```python
from build123d import *

# Parameters (mm, degrees)
SKETCH1_W                   = 173.0375
SKETCH1_H                   = 114.3
BOSS_EXTRUDE1_DEPTH         = 3.175
SKETCH3_R                   = 3.175
SKETCH3_R_2                 = 3.7703125
CUT_EXTRUDE1_DEPTH          = 4.175
F_6_CLEARANCE_HOLE1_D       = 4.3053
F_2_CLEARANCE_HOLE1_D       = 2.7051
SKETCH8_W                   = 58.74
SKETCH8_H                   = 26.99
CUT_EXTRUDE2_DEPTH          = 4.175
F_3_0_213_DIAMETER_HOLE1_D  = 5.4102
F_3_0_3_DIAMETER_HOLE1_D    = 3
FILLET1_R                   = 1.27
FILLET2_R                   = 2.54
F_1_4_CLEARANCE_HOLE1_D     = 7.14248
F_1_4_CLEARANCE_HOLE1_DEPTH = 3.175
CUT_EXTRUDE3_REACH          = 5.175
SKETCH14_W                  = 3.175
SKETCH14_H                  = 15.875
FILLET3_R                   = 1.5875
FILLET4_R                   = 2.54
CUT_EXTRUDE4_START          = -3.175
SKETCH15_W                  = 65.7
SKETCH15_H                  = 26.99
CUT_EXTRUDE4_DEPTH          = 3.175
CUT_EXTRUDE5_REACH          = 5.175
SKETCH16_R                  = 1.190625


with BuildPart() as part:
    # Sketch1 → Boss-Extrude1 (new body)
    with BuildSketch(Plane.XY):
        with Locations((25.118, -40.513)):
            Rectangle(SKETCH1_W, SKETCH1_H)
    extrude(amount=BOSS_EXTRUDE1_DEPTH)

    # Sketch3 → Cut-Extrude1 (cut, through all)
    with BuildSketch(Plane.XY.offset(3.175)):
        with Locations((100.302, -26.543)):
            Circle(SKETCH3_R)
        with Locations((99.413, -51.6255)):
            Circle(SKETCH3_R_2)
        with Locations((-47.907, -51.6255)):
            Circle(SKETCH3_R_2)
        with Locations((-47.907, -6.5405)):
            Circle(SKETCH3_R_2)
    extrude(amount=-CUT_EXTRUDE1_DEPTH, mode=Mode.SUBTRACT)

    # #6 Clearance Hole1 (through all)
    with Locations(Plane.XY.offset(3.175)):
        with Locations((18.387, 10.287), (-56.162, -40.894), (106.398, -40.894), (18.387, -91.313)):
            Hole(F_6_CLEARANCE_HOLE1_D / 2)

    # #2 Clearance Hole1 (through all)
    with Locations(Plane.XY.offset(3.175)):
        with Locations((26.788, 12.7), (89.488, 12.7), (89.488, -18.6), (26.788, -18.6)):
            Hole(F_2_CLEARANCE_HOLE1_D / 2)

    # Sketch8 → Cut-Extrude2 (cut, through all)
    with BuildSketch(Plane.XY.offset(3.175)):
        with Locations((58.138, -3.125)):
            Rectangle(SKETCH8_W, SKETCH8_H)
        Polygon((14.64685, 6.54685), (14.64685, 10.287), (-41.367, 10.287), (-41.367, -13.0805), (-55.05075, -13.0805), (-55.05075, -35.56635), (-50.83435, -35.56635), (-50.83435, -45.0855), (-41.367, -45.0855), (-41.367, -58.1655), (-55.05075, -58.1655), (-55.05075, -91.313), (13.05935, -91.313), (13.05935, -88.138), (105.28675, -88.138), (105.28675, -58.1655), (92.658, -58.1655), (92.658, -45.0855), (101.07035, -45.0855), (101.07035, -32.150898303), (92.658, -32.150898303), (92.658, -23.12755), (22.26045, -23.12755), (22.26045, 6.54685), align=None)
    extrude(amount=-CUT_EXTRUDE2_DEPTH, mode=Mode.SUBTRACT)

    # #3 (0.213) Diameter Hole1 (through all)
    with Locations(Plane(origin=(18.387, 10.287, 3.175), x_dir=(1, 0, 0), z_dir=(0, 0, 1))):
        with Locations((0, 0), (-74.549, -51.181), (0, -101.6), (88.011, -51.181)):
            Hole(F_3_0_213_DIAMETER_HOLE1_D / 2)

    # Ø3.0 (3) Diameter Hole1 (through all)
    with Locations(Plane.XY.offset(3.175)):
        with Locations((26.788, 12.7), (89.488, 12.7), (89.488, -18.6), (26.788, -18.6)):
            Hole(F_3_0_3_DIAMETER_HOLE1_D / 2)

    # Fillet1
    fillet1_edges = [part.edges().sort_by_distance(p)[0] for p in [
        (14.64685, 10.287, 1.5875),
        (14.64685, 6.54685, 1.5875),
        (22.26045, 6.54685, 1.5875),
        (22.26045, -23.12755, 1.5875),
        (92.658, -23.12755, 1.5875),
        (92.658, -32.150898303, 1.5875),
        (101.07035, -32.150898303, 1.5875),
        (101.07035, -45.0855, 1.5875),
        (92.658, -45.0855, 1.5875),
        (92.658, -58.1655, 1.5875),
        (105.28675, -58.1655, 1.5875),
        (13.05935, -91.313, 1.5875),
        (-55.05075, -91.313, 1.5875),
        (-55.05075, -58.1655, 1.5875),
        (-41.367, -58.1655, 1.5875),
        (-41.367, -45.0855, 1.5875),
        (-50.83435, -45.0855, 1.5875),
        (-55.05075, -35.56635, 1.5875),
        (-55.05075, -13.0805, 1.5875),
        (-41.367, -13.0805, 1.5875),
        (-41.367, 10.287, 1.5875),
    ]]
    fillet(fillet1_edges, radius=FILLET1_R)

    # Fillet2
    fillet2_edges = [part.edges().sort_by_distance(p)[0] for p in [
        (13.05935, -88.138, 1.5875),
        (-50.83435, -35.56635, 1.5875),
        (111.63675, 16.637, 1.5875),
        (111.63675, -97.663, 1.5875),
        (-61.40075, -97.663, 1.5875),
        (-61.40075, 16.637, 1.5875),
    ]]
    fillet(fillet2_edges, radius=FILLET2_R)

    # 1/4 Clearance Hole1
    with Locations(Plane(origin=(0, 0, 0), x_dir=(-1, 0, 0), z_dir=(0, 0, -1))):
        with Locations((-102.7785, 10.287), (52.5425, 10.287)):
            Hole(F_1_4_CLEARANCE_HOLE1_D / 2, depth=F_1_4_CLEARANCE_HOLE1_DEPTH)

    # Sketch14 → Cut-Extrude3 (cut, up to next)
    with BuildSketch(Plane(origin=(0, 0, 0), x_dir=(-1, 0, 0), z_dir=(0, 0, -1)), mode=Mode.PRIVATE) as cut_extrude3_sk1:
        with Locations((-110.04925, 8.6995)):
            Rectangle(SKETCH14_W, SKETCH14_H)
    cut_extrude3_tool1 = extrude(cut_extrude3_sk1.sketch, amount=-CUT_EXTRUDE3_REACH, mode=Mode.PRIVATE) & part.part
    add(cut_extrude3_tool1.solids().sort_by_distance((110.04925, 8.6995, 0))[0], mode=Mode.SUBTRACT)
    # Sketch14 → Cut-Extrude3 (cut, up to next)
    with BuildSketch(Plane(origin=(0, 0, 0), x_dir=(-1, 0, 0), z_dir=(0, 0, -1)), mode=Mode.PRIVATE) as cut_extrude3_sk2:
        with Locations((59.81325, 8.6995)):
            Rectangle(SKETCH14_W, SKETCH14_H)
    cut_extrude3_tool2 = extrude(cut_extrude3_sk2.sketch, amount=-CUT_EXTRUDE3_REACH, mode=Mode.PRIVATE) & part.part
    add(cut_extrude3_tool2.solids().sort_by_distance((-59.81325, 8.6995, 0))[0], mode=Mode.SUBTRACT)

    # Fillet3
    fillet3_edges = [part.edges().sort_by_distance(p)[0] for p in [
        (108.46175, 0.762, 1.5875),
        (-58.22575, 0.762, 1.5875),
    ]]
    fillet(fillet3_edges, radius=FILLET3_R)

    # Fillet4
    fillet4_edges = [part.edges().sort_by_distance(p)[0] for p in [
        (111.63675, 0.762, 1.5875),
        (108.46175, 16.637, 1.5875),
        (-58.22575, 16.637, 1.5875),
        (-61.40075, 0.762, 1.5875),
    ]]
    fillet(fillet4_edges, radius=FILLET4_R)

    # Sketch15 → Cut-Extrude4 (cut)
    with BuildSketch(Plane(origin=(0, 0, 0), x_dir=(-1, 0, 0), z_dir=(0, 0, -1)).offset(CUT_EXTRUDE4_START)):
        with Locations((-58.138, -3.125)):
            Rectangle(SKETCH15_W, SKETCH15_H)
    extrude(amount=CUT_EXTRUDE4_DEPTH, mode=Mode.SUBTRACT)

    # Sketch16 → Cut-Extrude5 (cut, up to next)
    with BuildSketch(Plane(origin=(0, 0, 0), x_dir=(-1, 0, 0), z_dir=(0, 0, -1)), mode=Mode.PRIVATE) as cut_extrude5_sk1:
        with Locations((-98.142490655, -57.489441166)):
            Circle(SKETCH16_R)
    cut_extrude5_tool1 = extrude(cut_extrude5_sk1.sketch, amount=-CUT_EXTRUDE5_REACH, mode=Mode.PRIVATE) & part.part
    add(cut_extrude5_tool1.solids().sort_by_distance((98.142491, -57.489441, 0))[0], mode=Mode.SUBTRACT)
    # Sketch16 → Cut-Extrude5 (cut, up to next)
    with BuildSketch(Plane(origin=(0, 0, 0), x_dir=(-1, 0, 0), z_dir=(0, 0, -1)), mode=Mode.PRIVATE) as cut_extrude5_sk2:
        with Locations((49.177509345, -57.489441166)):
            Circle(SKETCH16_R)
    cut_extrude5_tool2 = extrude(cut_extrude5_sk2.sketch, amount=-CUT_EXTRUDE5_REACH, mode=Mode.PRIVATE) & part.part
    add(cut_extrude5_tool2.solids().sort_by_distance((-49.177509, -57.489441, 0))[0], mode=Mode.SUBTRACT)
    # Sketch16 → Cut-Extrude5 (cut, up to next)
    with BuildSketch(Plane(origin=(0, 0, 0), x_dir=(-1, 0, 0), z_dir=(0, 0, -1)), mode=Mode.PRIVATE) as cut_extrude5_sk3:
        with Locations((49.177509345, -12.404441166)):
            Circle(SKETCH16_R)
    cut_extrude5_tool3 = extrude(cut_extrude5_sk3.sketch, amount=-CUT_EXTRUDE5_REACH, mode=Mode.PRIVATE) & part.part
    add(cut_extrude5_tool3.solids().sort_by_distance((-49.177509, -12.404441, 0))[0], mode=Mode.SUBTRACT)


solid = part.part
```
For this review, take the finished solid that the model builds, in its own axes (mm). A direction names the side the tool comes from. Round coordinates to 2 decimals unless told otherwise and drop trailing zeros. Loops run counter-clockwise (first coordinate to the right, second up) from the corner with the lowest first, then second, coordinate; pieces in that order, holes last.
Q1. Mouldability with a two-part tool opening along X and no side actions: class faces 1 (the face through (58, -16.62, 2)), 2 (the face through (111.637, -49, 2)), 3 (the face through (24, 16.637, 2)) as +X half, -X half, draft (parallel to the pull), parting line (faces both ways), or undercut.
Result sheet:
face 1: undercut
face 2: +X half
face 3: draft
Q2. To check wall thickness, follow line 1 along Y through (x, z) = (81.5, 1.75); line 2 along X through (y, z) = (-1.5, 0.3); line 3 along X through (y, z) = (-40.5, 0.6). State the ranges of each line that lie inside material, in increasing order.
Result sheet:
line 1: y = -97.66 to -88.14, -23.13 to -16.62, 10.37 to 16.64
line 2: x = -61.4 to -41.37, 22.26 to 25.29, 90.99 to 111.63
line 3: x = -61.4 to -58.84, -53.49 to -50.83, 101.07 to 103.72, 109.07 to 111.64
Q3. Insertion check: pin 1 Ø1.4 at (x, y) = (-49.18, -57.49) entering from +Z (1 decimal). The pin has a flat end and moves straight along its axis. Give the tip position at first contact, or say it passes through.
Result sheet:
pin 1: passes through
Q4. Add section C-C on z = 0.7. Give the number of separate pieces and of enclosed holes in the cut face, plus the area to 3 significant figures.
Result sheet:
separate pieces: 1
enclosed holes: 16
area: 5,200 mm2
Q5. Add section A-A on x = 7. Write out the cut boundary in (y, z) (3 decimals).
Result sheet:
outline: (-97.663, 0) - (-91.313, 0) - (-91.313, 3.175) - (-97.663, 3.175) - close; (10.287, 0) - (16.637, 0) - (16.637, 3.175) - (10.287, 3.175) - close
Q6. Add section B-B on x = 44.5. Write out the cut boundary in (y, z) (3 decimals), plus the area to 3 significant figures.
Result sheet:
outline: (-97.663, 0) - (-88.138, 0) - (-88.138, 3.175) - (-97.663, 3.175) - close; (-23.128, 0) - (-16.62, 0) - (-16.62, 3.175) - (-23.128, 3.175) - close; (10.37, 0) - (16.637, 0) - (16.637, 3.175) - (10.37, 3.175) - close
area: 70.8 mm2
Q7. Machinability: for faces 4 (the face through (-55.051, -75, 2)), 5 (the face through (-61.401, -49, 2)), which of the approach directions +Z, -Z, +X, -X, +Y, -Y give a long, thin tool a straight path to every point of the face, cutting with its end or side? Answer none if there is none.
Result sheet:
face 4: +Z, -Z
face 5: +Z, -Z, -X, +Y, -Y
